```python
from build123d import *

# Parameters (mm, degrees)
F2_DEPTH = 15
F0_R     = 8
F3_DEPTH = 80
F4_SIZE  = 1.5


with BuildPart() as f2:
    # F1 (on face) → F2 (new body)
    with BuildSketch(Plane.XY):
        Polygon((14.062501, -5.824878), (14.062501, 5.824878), (5.824878, 14.062501), (-5.824878, 14.062501), (-14.062501, 5.824878), (-14.062501, -5.824878), (-5.824878, -14.062501), (5.824878, -14.062501), align=None)
    extrude(amount=F2_DEPTH)

    # F0 (on Top) → F3 (join)
    with BuildSketch(Plane.XY):
        Circle(F0_R)
    extrude(amount=-F3_DEPTH)

    # F4
    f4_edges = [f2.edges().sort_by_distance(p)[0] for p in [
        (0, -14.062501, 15),
        (9.94369, -9.94369, 15),
        (14.062501, 0, 15),
        (9.94369, 9.94369, 15),
        (0, 14.062501, 15),
        (-9.94369, 9.94369, 15),
        (-14.062501, 0, 15),
        (-9.94369, -9.94369, 15),
    ]]
    chamfer(f4_edges, length=F4_SIZE)


solid = f2.part
```
Can you work these out from the model? Positions are in its coordinate system, mm. A direction names the side the tool comes from. Give positions to 0.01 mm unless a question says otherwise; leave off trailing zeros. Order: outer loops, then holes, each group sorted by start corner. A loop starts at its lowest first (then second) coordinate and runs counter-clockwise, first axis right, second up. Notation, with made-up numbers: M 21,-31.5 L 39,-31.5 A18 ccw 39,-9.5 Z; hole C 70,16 d11. An arc over 180 degrees is marked long. Write item = value, one per line. Start each with the question number.
Q1. Suppose I cut it at C-C (z = -37). Write out the boundary of the cut face in (x, y), plus the area to 3 significant figures.
Q2. Will these pins go through, and if not, where does the flat tip stop? pin 1 Ø2 at (x, z) = (-8, -60.5) entering from -Y; pin 2 Ø1.5 at (x, z) = (9.5, -63.5) entering from +Y; pin 3 Ø10 at (x, z) = (-9, -33.5) entering from +Y; pin 4 Ø6 at (y, z) = (6.5, -68.5) entering from +X.
Q3. Suppose I cut it at D-D (x = 9.75). Write out the boundary of the cut face in (y, z), plus the area to 3 significant figures.
Q4. I need wall thicknesses on probe 1 along Z at (x, y) = (-2, 11.5); probe 2 along X at (y, z) = (5.5, -70); probe 3 along Y at (x, z) = (-0.5, -16). Which ranges of each line are inside material? Lowest first, please. Write a range as [from, to].
Q5. For faces 1 (the flat face through (-6, 6, 0)), 2 (the flat face through (0, -14.063, 7)), which set-ups out of +Z, -Z, +X, -X, +Y, -Y let a thin tool reach every point of the face, with its end or its side?
Q6. Suppose I cut it at A-A (y = 0). Write out the boundary of the cut face in (x, z).
Check result:
q1.outline = C 0,0 d16
q1.area = 201 mm2
q2.pin_1 = -3.87
q2.pin_2 = through
q2.pin_3 = 6.93
q2.pin_4 = 7.19
q3.outline = M -10.14,0 L 10.14,0 L 10.14,13.5 L 8.02,15 L -8.02,15 L -10.14,13.5 Z
q3.area = 301 mm2
q4.probe_1 = [0, 15]
q4.probe_2 = [-5.81, 5.81]
q4.probe_3 = [-7.98, 7.98]
q5.face_1 = -Z
q5.face_2 = +Z, -Z, +X, -X, -Y
q6.outline = M -14.06,0 L -8,0 L -8,-80 L 8,-80 L 8,0 L 14.06,0 L 14.06,13.5 L 12.56,15 L -12.56,15 L -14.06,13.5 Z
